Build history of the part. All positions in model axes, mm. Face numbers are marked on the shaded views. A direction names the side the tool comes from. Round coordinates to 2 decimals unless told otherwise and drop trailing zeros. Loops run counter-clockwise (first coordinate to the right, second up) from the corner with the lowest first, then second, coordinate; pieces in that order, holes last.
from build123d import *

# Parameters (mm, degrees)
F1_DEPTH     = 5
F3_DEPTH     = 5.001
F5_DEPTH     = 35
F6_T4_DEPTH  = 17.0072864353
F6_S5_R      = 12
F6_T6_DEPTH  = 11
F6_T7_DEPTH  = 30
F7_R         = 7.5
F8_DEPTH     = 5
F9_R         = 45.5
F10_DEPTH    = 3.5
F12_DEPTH    = 1.5
F14_DEPTH    = 3.5
F18_W        = 15
F18_H        = 15
F19_DEPTH    = 1.5010001
F20_DEPTH    = 5.0010001
F21_R        = 1.5
F22_DEPTH    = 3
F23_T1_DEPTH = 1.5
F23_T3_DEPTH = 11.4776669635
F24_R        = 1.5
F25_SIZE     = 1


# Not quite as in the source:
# - a fillet or chamfer that OpenCascade refuses, or shapes differently, is made with other operations: its cross-section is extruded or revolved along the edge and cut away or added
# - a feature names something its author has since deleted; it is built from what else it names


with BuildPart() as f1:
    # F0 (on Top) → F1 (new body)
    with BuildSketch(Plane.XY):
        Polygon((8.5036432176, -40), (-8.5036432176, -40), (-8.5036432176, -110), (0, -110), (8.5036432176, -110), align=None)
    extrude(amount=F1_DEPTH)

    # F2 (on face) → F3 (cut, through all)
    with BuildSketch(Plane.XY.offset(5)):
        with BuildLine():
            Line((-3.15, -67.75), (3.15, -67.75))
            Line((3.15, -67.75), (3.15, -63.4))
            ThreePointArc((3.15, -63.4), (0.75, -61), (3.15, -58.6))
            Line((3.15, -58.6), (3.15, -46.25))
            Line((3.15, -46.25), (-3.15, -46.25))
            Line((-3.15, -46.25), (-3.15, -50.6))
            ThreePointArc((-3.15, -50.6), (-0.75, -53), (-3.15, -55.4))
            Line((-3.15, -55.4), (-3.15, -67.75))
        make_face()
    extrude(amount=-F3_DEPTH, mode=Mode.SUBTRACT)

    # F4 (on face) → F5 (join)
    with BuildSketch(Plane.XZ.offset(110)):
        with BuildLine():
            ThreePointArc((8.5036432176, 5), (0, 8.5331202898), (-8.5036432176, 5))
            Line((-8.5036432176, 5), (8.5036432176, 5))
        make_face()
    extrude(amount=-F5_DEPTH)

    # F6: fillet of radius 5 on 3 edges, made by hand


with BuildPart() as f6_tool2:
    # F6_s3 → F6_t4 (new body)
    with BuildSketch(Plane.YZ.offset(-8.5036432176)):
        with BuildLine():
            ThreePointArc((-70, 5), (-73.5355339059, 6.4644660941), (-75, 10))
            Line((-75, 10), (-75, 5))
            Line((-75, 5), (-70, 5))
        make_face()
    extrude(amount=F6_T4_DEPTH)

    # F6_s5 → F6_t6 (intersect, symmetric)
    with BuildSketch(Plane.XZ.offset(72.5)):
        with Locations((0, -3.4668797102)):
            Circle(F6_S5_R)
    extrude(amount=F6_T6_DEPTH, both=True, mode=Mode.INTERSECT)


with BuildPart() as f1_1:
    add(f1.part)

    # F6_t1: union F6_tool2
    add(f6_tool2.part)

    # F6_s8 → F6_t7 (cut)
    with BuildSketch(Plane.XY.offset(-12.5)):
        with BuildLine():
            ThreePointArc((-8.5036432176, -105), (-7.0391771236, -108.5355339059), (-3.5036432176, -110))
            Line((-3.5036432176, -110), (-8.5036432176, -110))
            Line((-8.5036432176, -110), (-8.5036432176, -105))
        make_face()
        with BuildLine():
            ThreePointArc((8.5036432176, -105), (7.0391771236, -108.5355339059), (3.5036432176, -110))
            Line((3.5036432176, -110), (8.5036432176, -110))
            Line((8.5036432176, -110), (8.5036432176, -105))
        make_face()
    extrude(amount=F6_T7_DEPTH, mode=Mode.SUBTRACT)

    # F7 (on Top) → F8 (join)
    with BuildSketch(Plane.XY):
        with BuildLine():
            Line((-8.5036432176, 0), (-8.5036432176, -40))
            Line((-8.5036432176, -40), (8.5036432176, -40))
            Line((8.5036432176, -40), (8.5036432176, 0))
            Line((8.5036432176, 0), (8.5036432176, 10.8923699759))
            ThreePointArc((8.5036432176, 10.8923699759), (0, 7.2507186355), (-8.5036432176, 10.8923699759))
            Line((-8.5036432176, 10.8923699759), (-8.5036432176, 0))
        make_face()
        with BuildLine():
            ThreePointArc((11.7492813645, 19), (-4.3665727862, 29.9077337098), (-8.5036432176, 10.8923699759))
            ThreePointArc((-8.5036432176, 10.8923699759), (0, 7.2507186355), (8.5036432176, 10.8923699759))
            ThreePointArc((8.5036432176, 10.8923699759), (10.9077337098, 14.6334272138), (11.7492813645, 19))
        make_face()
        with Locations((0, 19)):
            Circle(F7_R, mode=Mode.SUBTRACT)
    extrude(amount=F8_DEPTH)

    # F9 (on face) → F10 (cut)
    with BuildSketch(Plane.XY.offset(5)):
        Circle(F9_R)
    extrude(amount=-F10_DEPTH, mode=Mode.SUBTRACT)

    # F11 (on Top) → F12 (join)
    with BuildSketch(Plane.XY):
        with BuildLine():
            ThreePointArc((-13.5, 0), (-32, 18.5), (-50.5, 0))
            ThreePointArc((-50.5, 0), (0, -50.5), (50.5, 0))
            ThreePointArc((50.5, 0), (32, 18.5), (13.5, 0))
            Line((13.5, 0), (-13.5, 0))
        make_face()
    extrude(amount=F12_DEPTH)

    # F13 (on face) → F14 (join)
    with BuildSketch(Plane.XY.offset(1.5)):
        with BuildLine():
            ThreePointArc((32.173358544, -32.173358544), (0, -45.5), (-32.173358544, -32.173358544))
            Line((-32.173358544, -32.173358544), (-35.7088924499, -35.7088924499))
            ThreePointArc((-35.7088924499, -35.7088924499), (0, -50.5), (35.7088924499, -35.7088924499))
            Line((35.7088924499, -35.7088924499), (32.173358544, -32.173358544))
        make_face()
    extrude(amount=F14_DEPTH)

    # F17: sweep along a path in F17_path
    with BuildLine(Plane(origin=(32.173358544, -32.173358544, 5), x_dir=(0, 1, 0), z_dir=(0, 0, 1))) as f17_path:
        ThreePointArc((0, 0), (-13.326641456, 32.173358544), (0, 64.346717088))
    # F16 (on face) → F17 (sweep)
    with BuildSketch(Plane(origin=(0, 0, 0), x_dir=(0.7071067812, 0.7071067812, 0), z_dir=(0.7071067812, -0.7071067812, 0))):
        Polygon((-43, 5), (-45.5, 5), (-45.5, 2.5), align=None)
    sweep(path=f17_path.line)

    # F18 (on face) → F19 (cut, through all)
    with BuildSketch(Plane.XY.offset(1.5)):
        with Locations((-32, 0)):
            Rectangle(F18_W, F18_H)
        with Locations((32, 0)):
            Rectangle(F18_W, F18_H)
    extrude(amount=-F19_DEPTH, mode=Mode.SUBTRACT)

    # F2 (on face) → F20 (cut, through all)
    with BuildSketch(Plane.XY.offset(5)):
        with BuildLine():
            Line((-3.15, -67.75), (3.15, -67.75))
            Line((3.15, -67.75), (3.15, -63.4))
            ThreePointArc((3.15, -63.4), (0.75, -61), (3.15, -58.6))
            Line((3.15, -58.6), (3.15, -46.25))
            Line((3.15, -46.25), (-3.15, -46.25))
            Line((-3.15, -46.25), (-3.15, -50.6))
            ThreePointArc((-3.15, -50.6), (-0.75, -53), (-3.15, -55.4))
            Line((-3.15, -55.4), (-3.15, -67.75))
        make_face()
    extrude(amount=-F20_DEPTH, mode=Mode.SUBTRACT)

    # F21 (on face) → F22 (join)
    with BuildSketch(Plane.XY.offset(1.5)):
        Circle(F21_R)
    extrude(amount=F22_DEPTH)

    # F23: fillet of radius 3 on 16 edges, made by hand

    # F23_s2 → F23_t1 (join)
    with BuildSketch(Plane.XY):
        with BuildLine():
            ThreePointArc((-10.710331144, 0), (-12.6780946011, 0.7355117627), (-13.6809826122, 2.5813953488))
            ThreePointArc((-13.6809826122, 2.5813953488), (-13.5453011177, 1.2938659758), (-13.5, 0))
            Line((-13.5, 0), (-10.710331144, 0))
        make_face()
        with BuildLine():
            ThreePointArc((13.6809826122, 2.5813953488), (12.6780946011, 0.7355117627), (10.710331144, 0))
            Line((10.710331144, 0), (13.5, 0))
            ThreePointArc((13.5, 0), (13.5453011177, 1.2938659758), (13.6809826122, 2.5813953488))
        make_face()
        with BuildLine():
            ThreePointArc((39.5, -4.5), (38.6213203436, -6.6213203436), (36.5, -7.5))
            Line((36.5, -7.5), (39.5, -7.5))
            Line((39.5, -7.5), (39.5, -4.5))
        make_face()
        with BuildLine():
            ThreePointArc((24.5, -4.5), (25.3786796564, -6.6213203436), (27.5, -7.5))
            Line((27.5, -7.5), (24.5, -7.5))
            Line((24.5, -7.5), (24.5, -4.5))
        make_face()
        with BuildLine():
            ThreePointArc((24.5, 4.5), (25.3786796564, 6.6213203436), (27.5, 7.5))
            Line((27.5, 7.5), (24.5, 7.5))
            Line((24.5, 7.5), (24.5, 4.5))
        make_face()
        with BuildLine():
            ThreePointArc((36.5, 7.5), (38.6213203436, 6.6213203436), (39.5, 4.5))
            Line((39.5, 4.5), (39.5, 7.5))
            Line((39.5, 7.5), (36.5, 7.5))
        make_face()
        with BuildLine():
            ThreePointArc((-27.5, 7.5), (-25.3786796564, 6.6213203436), (-24.5, 4.5))
            Line((-24.5, 4.5), (-24.5, 7.5))
            Line((-24.5, 7.5), (-27.5, 7.5))
        make_face()
        with BuildLine():
            ThreePointArc((-36.5, -7.5), (-38.6213203436, -6.6213203436), (-39.5, -4.5))
            Line((-39.5, -4.5), (-39.5, -7.5))
            Line((-39.5, -7.5), (-36.5, -7.5))
        make_face()
        with BuildLine():
            ThreePointArc((-27.5, -7.5), (-25.3786796564, -6.6213203436), (-24.5, -4.5))
            Line((-24.5, -4.5), (-24.5, -7.5))
            Line((-24.5, -7.5), (-27.5, -7.5))
        make_face()
        with BuildLine():
            ThreePointArc((-39.5, 4.5), (-38.6213203436, 6.6213203436), (-36.5, 7.5))
            Line((-36.5, 7.5), (-39.5, 7.5))
            Line((-39.5, 7.5), (-39.5, 4.5))
        make_face()
        with BuildLine():
            ThreePointArc((11.5036432176, 0), (9.3823228741, 0.8786796564), (8.5036432176, 3))
            Line((8.5036432176, 3), (8.5036432176, 0))
            Line((8.5036432176, 0), (11.5036432176, 0))
        make_face()
        with BuildLine():
            ThreePointArc((-8.5036432176, 3), (-9.3823228741, 0.8786796564), (-11.5036432176, 0))
            Line((-11.5036432176, 0), (-8.5036432176, 0))
            Line((-8.5036432176, 0), (-8.5036432176, 3))
        make_face()
        with BuildLine():
            ThreePointArc((-9.163805174, 11.6467498809), (-8.6734917967, 10.7643189961), (-8.5036432176, 9.7692094873))
            Line((-8.5036432176, 9.7692094873), (-8.5036432176, 10.8923699759))
            ThreePointArc((-8.5036432176, 10.8923699759), (-8.8417733192, 11.2625160968), (-9.163805174, 11.6467498809))
        make_face()
        with BuildLine():
            ThreePointArc((8.5036432176, 9.7692094873), (8.6734917967, 10.7643189961), (9.163805174, 11.6467498809))
            ThreePointArc((9.163805174, 11.6467498809), (8.8417733192, 11.2625160968), (8.5036432176, 10.8923699759))
            Line((8.5036432176, 10.8923699759), (8.5036432176, 9.7692094873))
        make_face()
    extrude(amount=F23_T1_DEPTH)

    # F23_s4 → F23_t3 (cut)
    with BuildSketch(Plane.XY.offset(1.5)):
        with BuildLine():
            ThreePointArc((33.382302863, -37.8928998041), (34.3976980488, -35.7366206113), (33.5205161058, -33.5205161058))
            Line((33.5205161058, -33.5205161058), (35.7088924499, -35.7088924499))
            ThreePointArc((35.7088924499, -35.7088924499), (34.5628527392, -36.8192777024), (33.382302863, -37.8928998041))
        make_face()
        with BuildLine():
            ThreePointArc((-33.382302863, -37.8928998041), (-34.3976980488, -35.7366206113), (-33.5205161058, -33.5205161058))
            Line((-33.5205161058, -33.5205161058), (-35.7088924499, -35.7088924499))
            ThreePointArc((-35.7088924499, -35.7088924499), (-34.5628527392, -36.8192777024), (-33.382302863, -37.8928998041))
        make_face()
    extrude(amount=F23_T3_DEPTH, mode=Mode.SUBTRACT)

    # F24
    f24_edges = [f1_1.edges().sort_by_distance(p)[0] for p in [
        (-1.5, 0, 4.5),
    ]]
    fillet(f24_edges, radius=F24_R)

    # F25
    f25_edges = [f1_1.edges().sort_by_distance(p)[0] for p in [
        (21.769872, -45.566684, 5),
        (-21.769872, -45.566684, 5),
        (-34.397698, -35.736621, 5),
        (-31.963054, -31.963054, 5),
        (31.963054, -31.963054, 5),
        (34.397698, -35.736621, 5),
    ]]
    chamfer(f25_edges, length=F25_SIZE)


solid = f1_1.part
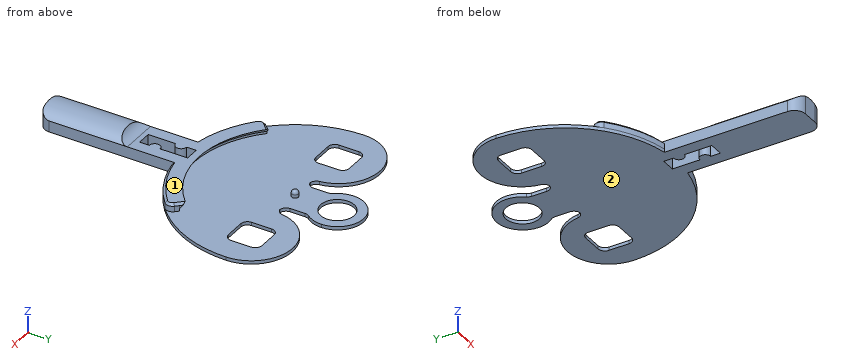
(1) Slice it at B-B on y = -19.5. List the corners of the cut face in (x, z), plus the area to 3 significant figures.
Responses:
outline: (-46.58, 0) - (46.58, 0) - (46.58, 1.5) - (-46.58, 1.5) - close
area: 140 mm2
(2) Which spindle directions (+Z, -Z, +X, -X, +Y, -Y) get a long thin tool onto all of the face, cutting with end or side? Do the marked faces 1 and 2. Say none if no direction does.
Responses:
face 1: +Z, +X, -X, +Y
face 2: -Z, +X, -X, +Y, -Y
(3) Pin check, flat tips, straight feed: P1, Ø6, axis at x = 2, y = -11.5, coming from the +Z side; P2, Ø2, axis at y = -89, z = 6.5, coming from the -X side; P3, Ø0.8, axis at y = 7.5, z = 0.5, coming from the -X side; P4, Ø2, axis at x = 7, y = -44.5, coming from the -Z side. Stop position of each tip, or through.
Responses:
P1: stops at z = 1.5
P2: stops at x = -7.97
P3: stops at x = -49.08
P4: stops at z = 0
(4) Probe line 1 (Y direction, x = 0, z = 0.9); line 2 (X direction, y = 19, z = 0.9); line 3 (X direction, y = -61, z = 3). List the from-to ranges inside material, lowest first.
Responses:
line 1: y = -110 to -67.75, -46.25 to 11.5, 26.5 to 30.75
line 2: x = -11.75 to -7.5, 7.5 to 11.75
line 3: x = -8.5 to -3.15, 0.75 to 8.5
(5) Slice it at A-A on y = -61. List the corners of the cut face in (x, z).
Responses:
outline: (-8.5, 0) - (-3.15, 0) - (-3.15, 5) - (-8.5, 5) - close; (0.75, 0) - (8.5, 0) - (8.5, 5) - (0.75, 5) - close
